Source: CAD feature listing. Evaluate the final solid. Frame: model axes, mm. A direction names the side the tool comes from. Coordinates: 2 decimals unless noted, no trailing zeros. Order: outer loops, then holes, each group sorted by start corner. A loop starts at its lowest first (then second) coordinate and runs counter-clockwise, first axis right, second up.
```python
from build123d import *

# Parameters (mm, degrees)
F1_DEPTH = 304.8
F2_R     = 0.508
F3_R     = 3.683


with BuildPart() as f1:
    # F0 (on Front) → F1 (new body)
    with BuildSketch(Plane.XZ):
        Polygon((-3.175, 0), (0, 0), (0, 38.1), (-38.1, 38.1), (-38.1, 28.575), (-23.116228, 28.575), (-23.116228, 16.091942), (-19.941228, 16.091942), (-19.941228, 31.75), (-34.925, 31.75), (-34.925, 34.925), (-3.175, 34.925), align=None)
    extrude(amount=-F1_DEPTH)

    # F2
    f2_edges = [f1.edges().sort_by_distance(p)[0] for p in [
        (-34.925, 152.4, 31.75),
        (-34.925, 152.4, 34.925),
        (-3.175, 152.4, 34.925),
        (-23.116228, 152.4, 28.575),
    ]]
    fillet(f2_edges, radius=F2_R)

    # F3
    f3_edges = [f1.edges().sort_by_distance(p)[0] for p in [
        (-38.1, 152.4, 38.1),
        (0, 152.4, 38.1),
        (-19.941228, 152.4, 31.75),
        (-38.1, 152.4, 28.575),
    ]]
    fillet(f3_edges, radius=F3_R)


solid = f1.part
```
1. Draft query along X for faces 1 (the flat face through (-23.116, 150, 22)), 2 (the flat face through (-3.175, 150, 17)), 3 (the flat face through (-21, 0, 26)). Return one class per face: +X half, -X half, draft (parallel to the pull), parting line (faces both ways), or undercut.
2. Section query A-A, the plane x = -31. Output: boundary loops of the cut face in (y, z) (3 decimals), plus the area to 3 significant figures.
3. Access query for faces 4 (the flat face through (-19.941, 150, 22)), 5 (the flat face through (-29, 150, 31.75)), 6 (the flat face through (-29, 150, 28.575)). Directions: +Z, -Z, +X, -X, +Y, -Y. A direction counts if a zero-diameter tool reaches every point of the face in a straight line with its end or side. Return the directions, or none.
4. Material intervals for line 1 along X through (y, z) = (60, 22) (3 decimals); line 2 along Z through (x, y) = (-28.5, 105) (3 decimals); line 3 along Z through (x, y) = (-6, 134) (3 decimals), sorted ascending.
5. Section query B-B, the plane z = 24.5. Output: boundary loops of the cut face in (x, y) (3 decimals).
6. Section query D-D, the plane z = 8. Output: boundary loops of the cut face in (x, y) (3 decimals).
7. Section query C-C, the plane y = 80.5. Output: boundary loops of the cut face in (x, z) (3 decimals).
8. Contact query for flat-ended pins moving along their axis: P1, Ø12, axis at x = -28.5, y = 126.5, coming from the -Z side; P2, Ø10.5, axis at y = 208, z = 16.5, coming from the -X side. Output: stop coordinate, or through.
Answer key:
1. face 1: -X half
1. face 2: undercut
1. face 3: draft
2. outline: (0, 28.575) - (304.8, 28.575) - (304.8, 31.75) - (0, 31.75) - close; (0, 34.925) - (304.8, 34.925) - (304.8, 38.1) - (0, 38.1) - close
2. area: 1,940 mm2
3. face 4: -Z, +Y, -Y
3. face 5: +Y, -Y
3. face 6: -Z, -X, +Y, -Y
4. line 1: x = -23.116 to -19.941, -3.175 to 0
4. line 2: z = 28.575 to 31.75, 34.925 to 38.1
4. line 3: z = 34.925 to 38.1
5. outline: (-23.116, 0) - (-19.941, 0) - (-19.941, 304.8) - (-23.116, 304.8) - close; (-3.175, 0) - (0, 0) - (0, 304.8) - (-3.175, 304.8) - close
6. outline: (-3.175, 0) - (0, 0) - (0, 304.8) - (-3.175, 304.8) - close
7. outline: (-38.1, 32.258) arc R3.683 ccw to (-34.417, 28.575) - (-23.624, 28.575) arc R0.508 cw to (-23.116, 28.067) - (-23.116, 16.092) - (-19.941, 16.092) - (-19.941, 28.067) arc R3.683 ccw to (-23.624, 31.75) - (-34.417, 31.75) arc R0.508 cw to (-34.925, 32.258) - (-34.925, 34.417) arc R0.508 cw to (-34.417, 34.925) - (-3.683, 34.925) arc R0.508 cw to (-3.175, 34.417) - (-3.175, 0) - (0, 0) - (0, 34.417) arc R3.683 ccw to (-3.683, 38.1) - (-34.417, 38.1) arc R3.683 ccw to (-38.1, 34.417) - close
8. P1: stops at z = 16.09
8. P2: stops at x = -23.12
